Can you work these out from the drawing? Everything is in mm from the part's minimum corner. Give positions to 0.01 mm unless a question says otherwise; leave off trailing zeros. Write each loop counter-clockwise with the first axis right and the second up, starting at its lowest first coordinate (ties: lowest second). Pieces come first, ordered by that corner, then holes. Notation, with made-up numbers: (68.25, 88) - (94.25, 88) arc R18 ccw to (94.25, 111) - close; hole circle Ø6 at (7, 60.5). An arc over 180 degrees is marked (long way). Write each question's results on one line, items separated by ' | '. Start each with the question number.
Item 1: Suppose I cut it at A-A on x = 25. List the corners of the cut face in (y, z) for me.
Item 2: Suppose I cut it at B-B on z = 10. List the corners of the cut face in (x, y) for me.
Item 3: Will these pins go through, and if not, where does the flat tip stop? P1, Ø1, axis at x = 15, z = 19.5, coming from the +Y side; P2, Ø10, axis at x = 33, z = 21.5, coming from the -Y side; P3, Ø6, axis at y = 19, z = 20, coming from the -X side.
Item 4: Please list where these lines run through material, in increasing order: line 1 along Y through (x, z) = (25, 7.5); line 2 along Z through (x, y) = (8, 30); line 3 along X through (y, z) = (30, 14.25).
Item 5: We'd pull the mould along Y, two halves only. Please class the marked faces 1, 2 and 3: +Y half, -Y half, draft (parallel to the pull), parting line (faces both ways), or undercut.
Item 6: Suppose I cut it at D-D on x = 4.5. List the corners of the cut face in (y, z) for me, then the cut area to 3 significant figures.
Item 7: Suppose I cut it at C-C on y = 42. List the corners of the cut face in (x, z) for me, then the cut area to 3 significant figures.
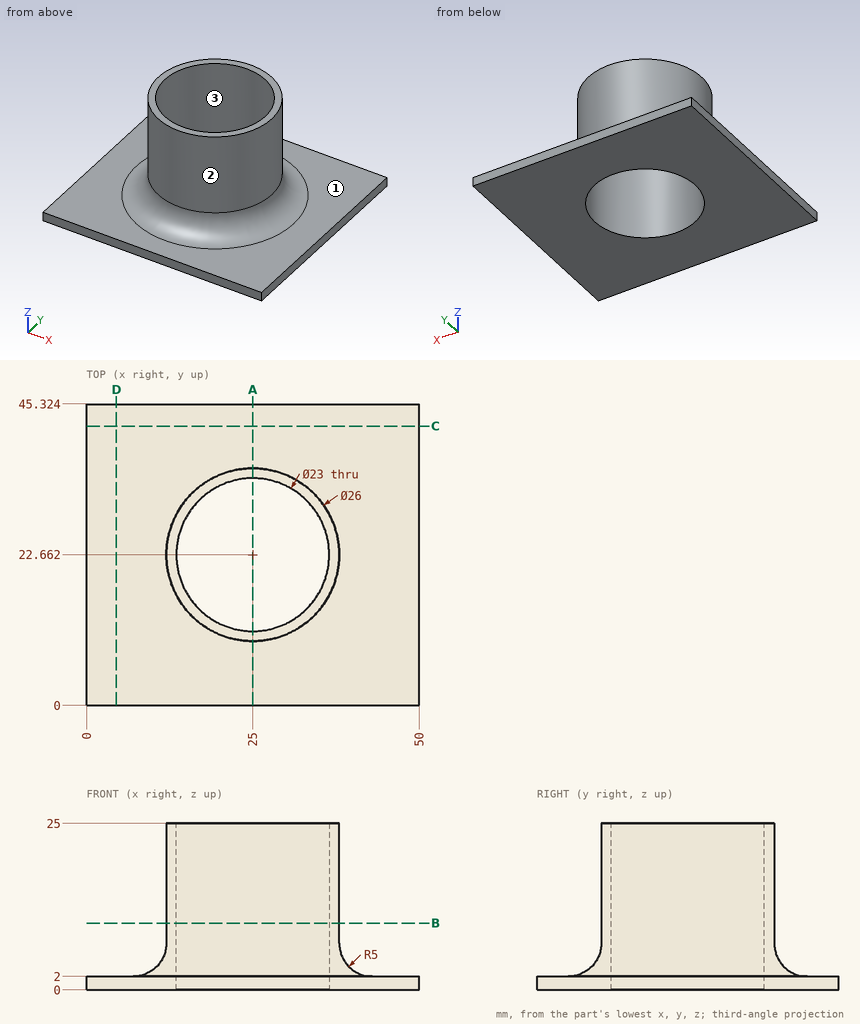
Checked values:
1) outline: (0, 0) - (11.16, 0) - (11.16, 25) - (9.66, 25) - (9.66, 7) arc R5 cw to (4.66, 2) - (0, 2) - close; (34.16, 0) - (45.32, 0) - (45.32, 2) - (40.66, 2) arc R5 cw to (35.66, 7) - (35.66, 25) - (34.16, 25) - close
2) outline: circle Ø26 at (25, 22.66); hole circle Ø23 at (25, 22.66)
3) P1: stops at y = 31.54 | P2: stops at y = 10.01 | P3: stops at x = 12.02
4) line 1: y = 9.66 to 11.16, 34.16 to 35.66 | line 2: z = 0 to 2 | line 3: x = 14.27 to 16.15, 33.85 to 35.73
5) face 1: draft | face 2: parting line | face 3: undercut
6) outline: (0, 0) - (45.32, 0) - (45.32, 2) - (0, 2) - close | area: 90.6 mm^2
7) outline: (0, 0) - (50, 0) - (50, 2) - (0, 2) - close | area: 100 mm^2
